Read the model definition and answer for the solid it produces. Units are mm, in the model's axes. A direction names the side the tool comes from. Give positions to 0.01 mm unless a question says otherwise; leave off trailing zeros. Loops run counter-clockwise (first coordinate to the right, second up) from the corner with the lowest first, then second, coordinate; pieces in that order, holes last. Notation, with made-up numbers: (75.25, 70) -> (97.25, 70) arc R13 ccw to (97.25, 74) -> close; hole circle Ø2 at (16, 51). An arc over 180 degrees is marked (long way). Write each question's results on one line, items separated by ' | '. Start each with the question number.
Item 1: Section A-A on x = 47.5 is taken. Write down the section's boundary in (y, z), and give its area (4 significant figures).
Item 2: Determine the mould class of faces 1 (the flat face through (50.5, 6, 13)), 2 (the flat face through (25, 0, 13)), 3 (the flat face through (0, 6, 13)) for opening direction X: +X half, -X half, draft (parallel to the pull), parting line (faces both ways), or undercut.
Item 3: Which of the six approach directions +Z, -Z, +X, -X, +Y, -Y give full straight-line access (tool end or side, diameter ignored) to faces 4 (the flat face through (25, 7, 25)), 5 (the flat face through (25, 7, 2)), 6 (the flat face through (25, 10, 0))?
Item 4: Section C-C on z = 2.5 is taken. Write down the section's boundary in (x, y).
Item 5: Find the intervals of material crossed by line 1 (Y direction, x = 30, z = 2.5); line 2 (Z direction, x = 45, y = 3.5), in increasing order.
Item 6: Section B-B on y = 4 is taken. Write down the section's boundary in (x, z).
Item 7: This flat-tipped pin is pushed along its axis until it touches: P1, Ø4, axis at x = 35.5, z = 25.5, coming from the -Y side. Where does it stop, or does it pass through?
```python
from build123d import *

# Parameters (mm, degrees)
BOX002002_W     = 50.5
BOX002002_H     = 7
BOX002002_DEPTH = 19.5
BOX002003_W     = 50.5
BOX002003_H     = 6
BOX002003_DEPTH = 27


with BuildPart() as f_7segment:
    # Box002002 → Box002002 (new body)
    with BuildSketch(Plane.XY.offset(3.7)):
        with Locations((25.25, 3.5)):
            Rectangle(BOX002002_W, BOX002002_H)
    extrude(amount=BOX002002_DEPTH)


with BuildPart() as f_7segmentbackpack:
    # Box002003 → Box002003 (new body)
    with BuildSketch(Plane(origin=(0, 7, 0), x_dir=(1, 0, 0), z_dir=(0, 0, 1))):
        with Locations((25.25, 3)):
            Rectangle(BOX002003_W, BOX002003_H)
    extrude(amount=BOX002003_DEPTH)

    # Fusion: union 7Segment
    add(f_7segment.part)


solid = f_7segmentbackpack.part
```
Findings:
1) outline: (0, 3.7) -> (7, 3.7) -> (7, 0) -> (13, 0) -> (13, 27) -> (7, 27) -> (7, 23.2) -> (0, 23.2) -> close | area: 298.5 mm2
2) face 1: +X half | face 2: draft | face 3: -X half
3) face 4: +Z, +X, -X, -Y | face 5: -Z, +X, -X, -Y | face 6: -Z, +X, -X, +Y, -Y
4) outline: (0, 7) -> (50.5, 7) -> (50.5, 13) -> (0, 13) -> close
5) line 1: 7 to 13 | line 2: 3.7 to 23.2
6) outline: (0, 3.7) -> (50.5, 3.7) -> (50.5, 23.2) -> (0, 23.2) -> close
7) P1: y = 7
